Could you check a few things on this model? Use its own coordinates, in mm. A direction names the side the tool comes from. Coordinates: 2 decimals unless noted, no trailing zeros. Loops run counter-clockwise (first coordinate to the right, second up) from the corner with the lowest first, then second, coordinate; pieces in that order, holes last.
from build123d import *

# Parameters (mm, degrees)
SKETCH1_R           = 0.75
SKETCH1_R_2         = 2.625
BOSS_EXTRUDE1_DEPTH = 3
VARFILLET1_START    = 9
VARFILLET1_DEPTH    = 27
CUT_EXTRUDE1_REACH  = 38.963
SKETCH2_R           = 10.5


with BuildPart() as part:
    # Sketch1 → Boss-Extrude1 (new body)
    with BuildSketch(Plane.XY):
        with BuildLine():
            Line((-6, 10), (-6, 0))
            ThreePointArc((-6, 0), (0, -6), (6, 0))
            Line((6, 0), (6, 35))
            Line((6, 35), (-11.5, 35))
            Line((-11.5, 35), (-11.5, 10))
            Line((-11.5, 10), (-6, 10))
        make_face()
        with Locations((1, 27.5)):
            Circle(SKETCH1_R, mode=Mode.SUBTRACT)
        Circle(SKETCH1_R_2, mode=Mode.SUBTRACT)
    extrude(amount=BOSS_EXTRUDE1_DEPTH)

    # VarFillet1: read off the stored shape, not the designer's step
    # VarFillet1 outline → VarFillet1 (cut)
    with BuildSketch(Plane(origin=(0, 0, 0), x_dir=(1, 0, 0), z_dir=(0, 1, 0)).offset(VARFILLET1_START)):
        with BuildLine():
            Line((-11.5, 0), (-11.5, -1))
            add(Edge.make_bspline(
                [(-11.5, -1), (-11.5, 0), (-10.5, 0)],
                knots=[0, 0, 0, 1, 1, 1], degree=2, weights=[1, 0.707106781, 1]))
            Line((-10.5, 0), (-11.5, 0))
        make_face()
        with BuildLine():
            add(Edge.make_bspline(
                [(-10.5, -3), (-11.5, -3), (-11.5, -2)],
                knots=[0, 0, 0, 1, 1, 1], degree=2, weights=[1, 0.707106781, 1]))
            Line((-11.5, -2), (-11.5, -3))
            Line((-11.5, -3), (-10.5, -3))
        make_face()
    extrude(amount=VARFILLET1_DEPTH, mode=Mode.SUBTRACT)

    # Sketch2 → Cut-Extrude1 (cut, up to next)
    with BuildSketch(Plane.XY.offset(3), mode=Mode.PRIVATE) as cut_extrude1_sk1:
        with Locations((-14, 22.5)):
            Circle(SKETCH2_R)
    cut_extrude1_tool1 = extrude(cut_extrude1_sk1.sketch, amount=-CUT_EXTRUDE1_REACH, mode=Mode.PRIVATE) & part.part
    add(cut_extrude1_tool1.solids().sort_by_distance((-14, 22.5, 3))[0], mode=Mode.SUBTRACT)


solid = part.part
(1) Imagine slicing it at C-C, the plane x = 1. Write out the boundary of the cut face in (y, z).
Answers:
outline: (-5.92, 0) - (-2.43, 0) - (-2.43, 3) - (-5.92, 3) - close; (2.43, 0) - (26.75, 0) - (26.75, 3) - (2.43, 3) - close; (28.25, 0) - (35, 0) - (35, 3) - (28.25, 3) - close
(2) Imagine slicing it at A-A, the plane x = -4.25. Write out the boundary of the cut face in (y, z).
Answers:
outline: (-4.24, 0) - (18.6, 0) - (18.6, 3) - (-4.24, 3) - close; (26.4, 0) - (35, 0) - (35, 3) - (26.4, 3) - close
(3) For pin 1 (0.9 mm diameter, centred on x = 1, y = 27.5, fed in from +Z); pin 2 (0.9 mm diameter, centred on x = -9.5, z = 1.5, fed in from -Y); pin 3 (0.9 mm diameter, centred on y = 6, z = 1, fed in from -X), each with a flat end and sliding along its axis, tell me the tip position at first contact or that it passes through.
Answers:
pin 1: passes through
pin 2: stops at y = 10
pin 3: stops at x = -6
(4) We'd pull the mould along Y, two halves only. Please class faces 1 (the face through (-1, 15, 3)), 2 (the face through (0, -6, 1)), 3 (the face through (2.5, 0.8, 1.5)): +Y half, -Y half, draft (parallel to the pull), parting line (faces both ways), or undercut.
Answers:
face 1: draft
face 2: -Y half
face 3: undercut
(5) Imagine slicing it at D-D, the plane y = 4.5. Write out the boundary of the cut face in (x, z), and give its area (3 significant figures).
Answers:
outline: (-6, 0) - (6, 0) - (6, 3) - (-6, 3) - close
area: 36.0 mm2
(6) I need wall thicknesses on probe 1 along Y at (x, z) = (1, 2.25); probe 2 along X at (y, z) = (22.5, 0.7); probe 3 along Y at (x, z) = (-5.5, 2.6). Which ranges of each line are inside material? Lowest first, please.
Answers:
probe 1: y = -5.92 to -2.43, 2.43 to 26.75, 28.25 to 35
probe 2: x = -3.5 to 6
probe 3: y = -2.4 to 16.34, 28.66 to 35
(7) Which directions (+Z, -Z, +X, -X, +Y, -Y) give clear straight access to the entire face, cutting with the end or side of a thin tool? Please do faces 4 (the face through (-11.5, 11.2, 1.5)), 5 (the face through (-9, 10, 1)).
Answers:
face 4: +Z, -Z, -X, +Y, -Y
face 5: +Z, -Z, -X, -Y
(8) Imagine slicing it at B-B, the plane y = 27.5. Write out the boundary of the cut face in (x, z), and give its area (3 significant figures).
Answers:
outline: (-4.77, 0) - (0.25, 0) - (0.25, 3) - (-4.77, 3) - close; (1.75, 0) - (6, 0) - (6, 3) - (1.75, 3) - close
area: 27.8 mm2
